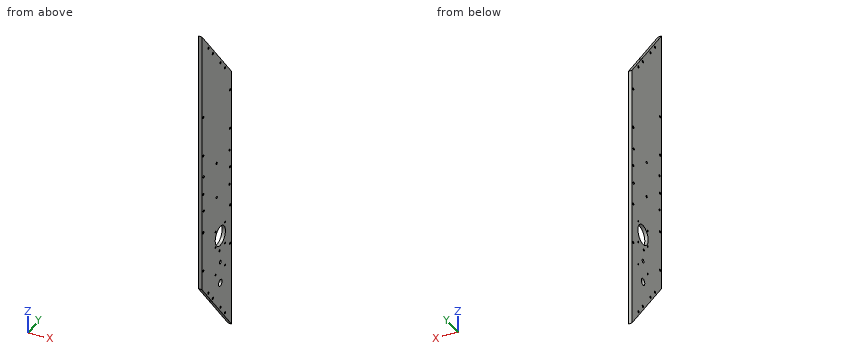
from build123d import *

# Parameters (mm, degrees)
BOSS_EXTRUDE1_DEPTH          = 4.7625
SKETCH2_R                    = 2.5
SKETCH2_R_2                  = 1.51
SKETCH2_R_3                  = 14
SKETCH2_R_4                  = 4.7625
GEARBOX_WITH_SLIP_FITS_DEPTH = 412.602247496
SKETCH5_R                    = 1.59385
CUT_EXTRUDE1_DEPTH           = 412.602247496
F_2_CLEARANCE_HOLE1_D        = 2.4384
F_4_CLEARANCE_HOLE2_D        = 3.2639
F_4_CLEARANCE_HOLE1_D        = 3.2639
F_4_CLEARANCE_HOLE1_DEPTH    = 4.826
F_4_CLEARANCE_HOLE1_TIP      = 0.980574487


with BuildPart() as part:
    # Sketch1 → Boss-Extrude1 (new body)
    with BuildSketch(Plane(origin=(0, 0, 0), x_dir=(0, 0, -1), z_dir=(1, 0, 0))):
        Polygon((33.297595377, -40.64), (312.697595377, -40.64), (345.995190754, -12.7), (409.563327383, 40.64), (312.697595377, 40.64), (33.297595377, 40.64), (0, 12.7), (-63.568136629, -40.64), align=None)
    extrude(amount=BOSS_EXTRUDE1_DEPTH)

    # Sketch2 → Gearbox (with Slip fits) (cut, through all)
    with BuildSketch(Plane(origin=(4.7625, 0, 0), x_dir=(0, 0, -1), z_dir=(1, 0, 0))):
        with Locations((300.047997385, 10.000000066)):
            Circle(SKETCH2_R)
        with Locations((282.21469668, 8.000000066)):
            Circle(SKETCH2_R_2)
        with Locations((261.047997385, 10.000000066)):
            Circle(SKETCH2_R_3)
        with Locations((331.004197385, 10.000000066)):
            Circle(SKETCH2_R_4)
    extrude(amount=-GEARBOX_WITH_SLIP_FITS_DEPTH, mode=Mode.SUBTRACT)

    # Sketch5 → Cut-Extrude1 (cut, through all)
    with BuildSketch(Plane(origin=(4.7625, 0, 0), x_dir=(0, 0, -1), z_dir=(1, 0, 0))):
        with Locations((287.297595377, 36.83)):
            Circle(SKETCH5_R)
        with Locations((230.147595377, 36.83)):
            Circle(SKETCH5_R)
        with Locations((172.997595377, 36.83)):
            Circle(SKETCH5_R)
        with Locations((115.847595377, 36.83)):
            Circle(SKETCH5_R)
        with Locations((58.697595377, 36.83)):
            Circle(SKETCH5_R)
        with Locations((58.697595377, -36.83)):
            Circle(SKETCH5_R)
        with Locations((115.847595377, -36.83)):
            Circle(SKETCH5_R)
        with Locations((172.997595377, -36.83)):
            Circle(SKETCH5_R)
        with Locations((230.147595377, -36.83)):
            Circle(SKETCH5_R)
        with Locations((287.297595377, -36.83)):
            Circle(SKETCH5_R)
    extrude(amount=-CUT_EXTRUDE1_DEPTH, mode=Mode.SUBTRACT)

    # #2 Clearance Hole1 (through all)
    with Locations(Plane(origin=(4.7625, 0, 0), x_dir=(0, 0, -1), z_dir=(1, 0, 0))):
        with Locations((248.047997385, 23.000000066), (279.047997385, 23.000000066), (271.047997455, -2.999999934), (248.047997385, -2.999999934), (312.047997385, 23.000000066), (312.047997385, -2.999999934)):
            Hole(F_2_CLEARANCE_HOLE1_D / 2)

    # #4 Clearance Hole2 (through all)
    with Locations(Plane(origin=(4.7625, 0, 0), x_dir=(0, 0, -1), z_dir=(1, 0, 0))):
        with Locations((147.597595377, 35.56), (198.397595377, 35.56), (198.397595377, -35.56), (147.597595377, -35.56), (147.597595377, 0), (198.397595377, 0)):
            Hole(F_4_CLEARANCE_HOLE2_D / 2)

    # #4 Clearance Hole1
    with Locations(Plane(origin=(4.7625, 0, 0), x_dir=(0, 0, -1), z_dir=(1, 0, 0))):
        with Locations((327.962613202, -22.8575274), (342.555759844, -10.612423436), (367.850547356, 10.612423436), (382.443693997, 22.8575274), (-36.448503243, -22.8575274), (-21.855356602, -10.612423436), (3.43943091, 10.612423436), (18.032577552, 22.8575274)):
            Hole(F_4_CLEARANCE_HOLE1_D / 2, depth=F_4_CLEARANCE_HOLE1_DEPTH)
            with Locations((0, 0, -(F_4_CLEARANCE_HOLE1_DEPTH + F_4_CLEARANCE_HOLE1_TIP / 2))):  # 118° drill point
                Cone(0, F_4_CLEARANCE_HOLE1_D / 2, F_4_CLEARANCE_HOLE1_TIP, mode=Mode.SUBTRACT)


solid = part.part
The model under review builds one solid part; all positions refer to its coordinate system, in mm. Coordinates: 2 decimals unless noted, no trailing zeros. Write each loop counter-clockwise with the first axis right and the second up, starting at its lowest first coordinate (ties: lowest second). Pieces come first, ordered by that corner, then holes. Notation, with made-up numbers: (43, -35.75) -> (98, -35.75) arc R17 cw to (98, -24.75) -> close; hole circle Ø6 at (18.25, 28.5). An arc over 180 degrees is marked (long way). Answer in a Markdown table with one row per item.
1. Clearance check with flat-ended pins moving along their axes: pin 1 Ø1.5 at (x, y) = (2.5, -8) entering from +Z; pin 2 Ø1.5 at (x, z) = (3, -27) entering from +Y (3 decimals). State where each tip first meets the part, or that it passes through.
Answers below:
| item | result |
|---|---|
| pin 1 | stops at z = 25.56 |
| pin 2 | stops at y = 35.985 |
2. We need section A-A, the plane x = 0.95. Give the number of separate pieces and of enclosed holes in the cut face, and give its area (3 significant figures).
Answers below:
| item | result |
|---|---|
| separate pieces | 1 |
| enclosed holes | 34 |
| area | 29,600 mm^2 |
3. We need section B-B, the plane z = -357.5. State the section outline as (x, y) points.
Answers below:
| item | result |
|---|---|
| outline | (0, -3.05) -> (4.76, -3.05) -> (4.76, 40.64) -> (0, 40.64) -> close |
4. Wall thickness on probe 1 along Y at (x, z) = (3.6, -172.5); probe 2 along Z at (x, y) = (4.55, -12); probe 3 along Z at (x, y) = (4.2, -2.5): over which ranges is each line inside the solid? List them lowest first. Write a range as [from, to].
Answers below:
| item | result |
|---|---|
| probe 1 | y = [-40.64, -38.34], [-35.32, 35.32], [38.34, 40.64] |
| probe 2 | z = [-346.83, -343.41], [-341.7, 21], [22.71, 29.44] |
| probe 3 | z = [-358.15, -313.16], [-310.94, -272.16], [-269.94, -267.35], [-254.74, -249.16], [-246.94, 18.11] |
